from build123d import *

# Parameters (mm, degrees)
SKETCH1_R           = 13
BOSS_EXTRUDE3_DEPTH = 6
SKETCH3_W           = 20
SKETCH3_H           = 6
BOSS_EXTRUDE4_DEPTH = 200
SKETCH5_W           = 20
SKETCH5_H           = 10
SKETCH5_R           = 3
BOSS_EXTRUDE5_DEPTH = 6


with BuildPart() as part:
    # Sketch1 → Boss-Extrude3 (new body)
    with BuildSketch(Plane.XY):
        with BuildLine():
            Line((77.458052403, 42.618499055), (77.458052403, 2.618499055))
            Line((77.458052403, 2.618499055), (27.458052403, 2.618499055))
            Line((27.458052403, 2.618499055), (27.458052403, 42.618499055))
            ThreePointArc((27.458052403, 42.618499055), (52.458052403, 67.618499055), (77.458052403, 42.618499055))
        make_face()
        with Locations((52.458052403, 42.618499055)):
            Circle(SKETCH1_R, mode=Mode.SUBTRACT)
    extrude(amount=BOSS_EXTRUDE3_DEPTH)

    # Sketch3 → Boss-Extrude4 (add)
    with BuildSketch(Plane.XZ.offset(-2.618499055)):
        with Locations((52.458052403, 3)):
            Rectangle(SKETCH3_W, SKETCH3_H)
    extrude(amount=BOSS_EXTRUDE4_DEPTH)

    # Sketch5 → Boss-Extrude5 (add)
    with BuildSketch(Plane.XY.offset(6)):
        with Locations((52.458052403, -202.381500945)):
            Rectangle(SKETCH5_W, SKETCH5_H)
        with Locations((52.458052403, -202.381500945)):
            Circle(SKETCH5_R, mode=Mode.SUBTRACT)
    extrude(amount=-BOSS_EXTRUDE5_DEPTH)


solid = part.part
Work out the finished part from the listing and answer in its coordinate system (mm). A direction names the side the tool comes from. Round coordinates to 2 decimals unless told otherwise and drop trailing zeros. Loops run counter-clockwise (first coordinate to the right, second up) from the corner with the lowest first, then second, coordinate; pieces in that order, holes last. Notation, with made-up numbers: M 25,-28.75 L 31,-28.75 A21 cw 31,-15.75 Z; hole C 79,40.25 d3. An arc over 180 degrees is marked long. One line per question, with ' | ' between items. Start each with the question number.
(1) A cutting plane is placed at A-A on x = 52. Write down the section's boundary in (y, z), plus the area to 3 significant figures.
(2) Find the intervals of material crossed by line 1 (Y direction, x = 55, z = 1.3); line 2 (Y direction, x = 50, z = 2.55); line 3 (X direction, y = -162, z = 3.9), in increasing order.
(3) A cutting plane is placed at B-B on y = 35.5. Write down the section's boundary in (x, z), plus the area to 3 significant figures.
(4) For a pull along Y with two mould halves and no side action, classify faces 1 (the face through (53.842, -205.043, 3.042)), 2 (the face through (27.458, 22, 3)), 3 (the face through (35, 2.618, 3)), 4 (the face through (42.14, 34.71, 2.96)) as released by +Y, released by -Y, zero draft, split by the parting line, or undercut.
(5) A tool of negligible diameter and unlimited length cuts with its end or side. For faces 5 (the face through (52, -37, 0)), 6 (the face through (42.458, -104, 3)), 7 (the face through (70, 2.618, 3)), from which of +Z, -Z, +X, -X, +Y, -Y can it reach the whole face along a straight path? Write none if from no direction.
(6) Flat-ended cylindrical pins translate along their axes: pin 1 Ø1.8 at (y, z) = (-87, 3) entering from +X; pin 2 Ø4 at (x, y) = (39.5, -38) entering from +Z; pin 3 Ø1.8 at (y, z) = (-77, 2) entering from -X. Find the tip coordinate at first contact, or state that the pin passes through.
(7) A cutting plane is placed at C-C on z = 3.4. Write down the section's boundary in (x, y).
(8) A cutting plane is placed at D-D on y = -63. Write down the section's boundary in (x, z).
Geometry check:
1) outline: M -207.38,0 L -205.35,0 L -205.35,6 L -207.38,6 Z; M -199.42,0 L 29.63,0 L 29.63,6 L -199.42,6 Z; M 55.61,0 L 67.61,0 L 67.61,6 L 55.61,6 Z | area: 1,460 mm²
2) line 1: y = -207.38 to -203.97, -200.79 to 29.87, 55.37 to 67.49 | line 2: y = -207.38 to -204.1, -200.66 to 29.85, 55.38 to 67.5 | line 3: x = 42.46 to 62.46
3) outline: M 27.46,0 L 41.58,0 L 41.58,6 L 27.46,6 Z; M 63.34,0 L 77.46,0 L 77.46,6 L 63.34,6 Z | area: 169 mm²
4) face 1: undercut | face 2: zero draft | face 3: released by -Y | face 4: undercut
5) face 5: -Z, +X, -X, +Y, -Y | face 6: +Z, -Z, -X, -Y | face 7: +Z, -Z, +X, -Y
6) pin 1: stops at x = 62.46 | pin 2: passes through | pin 3: stops at x = 42.46
7) outline: M 27.46,2.62 L 42.46,2.62 L 42.46,-207.38 L 62.46,-207.38 L 62.46,2.62 L 77.46,2.62 L 77.46,42.62 A25 ccw 27.46,42.62 Z; hole C 52.46,42.62 d26; hole C 52.46,-202.38 d6
8) outline: M 42.46,0 L 62.46,0 L 62.46,6 L 42.46,6 Z
